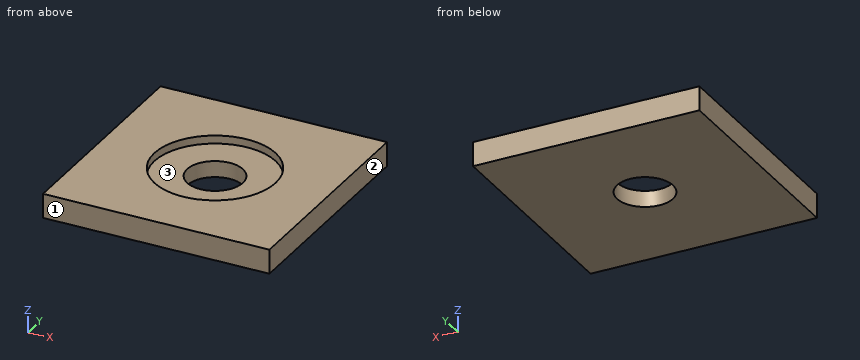
Autodesk Inventor part; units mm, degrees
ref_plane "YZ Plane" through (0, 0, 0) normal (1, 0, 0) x (0, 1, 0)
ref_plane "XZ Plane" through (0, 0, 0) normal (0, 1, 0) x (-1, 0, 0)
ref_plane "XY Plane" through (0, 0, 0) normal (0, 0, 1) x (1, 0, 0)
sketch "スケッチ1" plane through (0, 0, 0) normal (0, 0, 1) x (1, 0, 0)
  circle A0 centre (0, 0) radius 3.45
  circle A1 centre (0, 0) radius 7.5
  line L0 (-14, 14) -> (14, 14)
  line L1 (14, 14) -> (14, -14)
  line L2 (14, -14) -> (-14, -14)
  line L3 (-14, -14) -> (-14, 14)
  line L4 (-14, 14) -> (14, -14) construction
  line L5 (14, 14) -> (-14, -14) construction
  dimension "d0" = 6.9
  dimension "d1" = 15
  dimension "d2" = 28
  dimension "d3" = 28
extrude "押し出し1" add sketch "スケッチ1" along normal blind 3 contours L0 L1 L2 L3
extrude "押し出し2" add sketch "スケッチ1" along normal blind 2 contours A1
equation "\"d3\" = d2"
properties part number "baicPart"
The model under review builds one solid part; all positions refer to its coordinate system, in mm. Face numbers are marked on the shaded views. Round coordinates to 2 decimals unless told otherwise and drop trailing zeros. Loops run counter-clockwise (first coordinate to the right, second up) from the corner with the lowest first, then second, coordinate; pieces in that order, holes last. Notation, with made-up numbers: (-14, 59.5) - (8, 59.5) arc R21 cw to (8, 96.5) - close; hole circle Ø6 at (71, 30). An arc over 180 degrees is marked (long way). Use a Markdown table: item, result. Add a question column.
Q1. For probe 1 along Y at (x, z) = (0, 1.05); probe 2 along Y at (x, z) = (0, 2.45); probe 3 along Z at (x, y) = (-4.75, -3.75), list the stretches that pass through material, from the lowest coordinate up.
Q2. Add section D-D (x = -6.75). State the section outline as (y, z) points, plus the area to 3 significant figures.
Q3. Add section A-A (y = 0). State the section outline as (x, z) points, plus the area to 3 significant figures.
Q4. Insertion check: pin 1 Ø13.5 at (x, y) = (0, 0) entering from +Z; pin 2 Ø4 at (x, y) = (0, 0) entering from +Z. Each pin has a flat end and moves straight along its axis. Give the tip position at first contact, or say it passes through.
Q5. The part is to be moulded in two halves that separate along Y. For the marked faces 1, 2 and 3, say which applies: pulls with the +Y half, pulls with the -Y half, needs draft (parallel to the pull), parting line crosses it, or undercut.
Q6. Add section C-C (z = 1). State the section outline as (x, y) points.
Worked answers:
| question | item | result |
|---|---|---|
| 1 | probe 1 | -14 to -3.45, 3.45 to 14 |
| 1 | probe 2 | -14 to -7.5, 7.5 to 14 |
| 1 | probe 3 | 0 to 2 |
| 2 | outline | (-14, 0) - (14, 0) - (14, 3) - (3.27, 3) - (3.27, 2) - (-3.27, 2) - (-3.27, 3) - (-14, 3) - close |
| 2 | area | 77.5 mm² |
| 3 | outline | (-14, 0) - (-3.45, 0) - (-3.45, 2) - (-7.5, 2) - (-7.5, 3) - (-14, 3) - close; (3.45, 0) - (14, 0) - (14, 3) - (7.5, 3) - (7.5, 2) - (3.45, 2) - close |
| 3 | area | 55.2 mm² |
| 4 | pin 1 | z = 2 |
| 4 | pin 2 | through |
| 5 | face 1 | pulls with the -Y half |
| 5 | face 2 | needs draft |
| 5 | face 3 | undercut |
| 6 | outline | (-14, -14) - (14, -14) - (14, 14) - (-14, 14) - close; hole circle Ø6.9 at (0, 0) |
